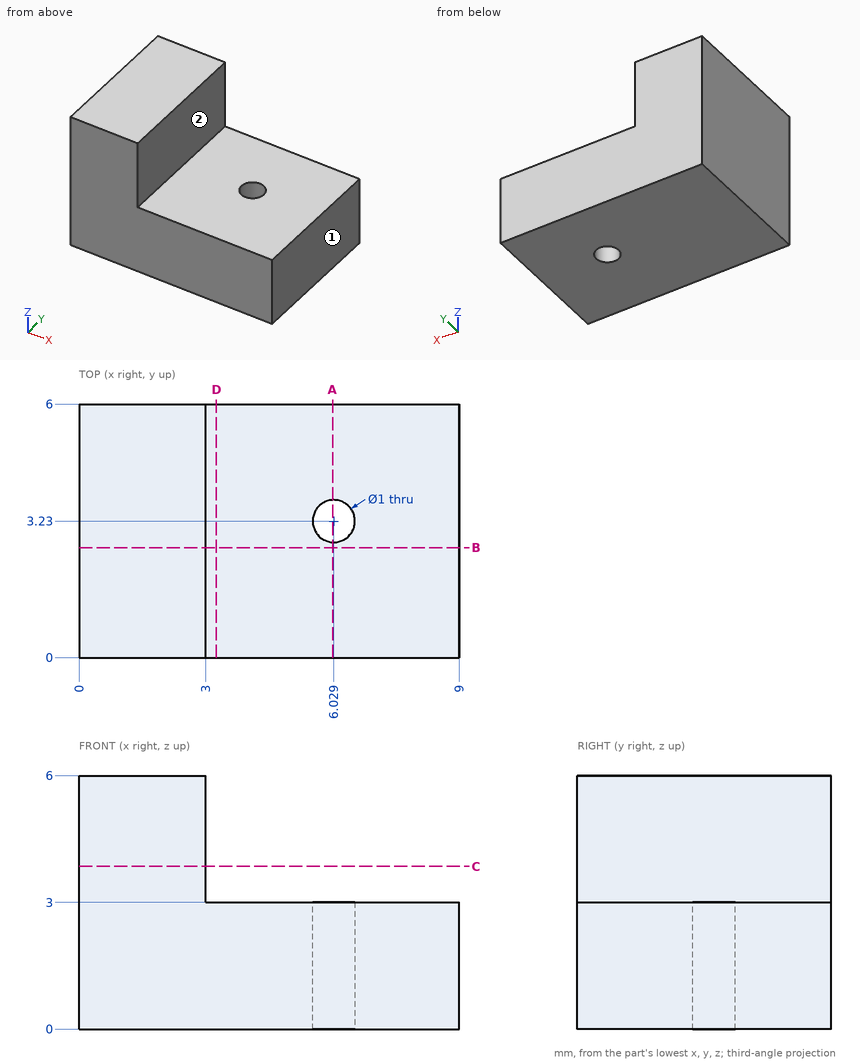
For this review, use the dimensioned drawing (mm, ordinates from the lowest corner) and the shaded views. A direction names the side the tool comes from. Round coordinates to 2 decimals unless told otherwise and drop trailing zeros. Order: outer loops, then holes, each group sorted by start corner. A loop starts at its lowest first (then second) coordinate and runs counter-clockwise, first axis right, second up. Notation, with made-up numbers: (62, -1) -> (116, -1) arc R26 cw to (116, 19) -> close; hole circle Ø9 at (-30, -18). An arc over 180 degrees is marked (long way). Write item = value, one per line. Start each with the question number.
Item 1: Clearance check with a flat-ended pin moving along its axis: pin 1 Ø3 at (x, y) = (6, 2.5) entering from +Z. State where the tip first meets the part, or that it passes through.
Item 2: For the marked faces 1 and 2, list the 3-axis set-ups (+Z, -Z, +X, -X, +Y, -Y) from which the entire face can be reached by the end or side of a thin tool; tool diameter is ignored.
Item 3: Consider section A-A on x = 6. Write out the cut boundary in (y, z).
Item 4: For line 1 along X through (y, z) = (4.2, 3.6); line 2 along X through (y, z) = (3.5, 0.6), list the stretches that pass through material, from the lowest coordinate up.
Item 5: Consider section B-B on y = 2.6. Write out the cut boundary in (x, z), plus the area to 3 significant figures.
Item 6: Consider section D-D on x = 3.25. Write out the cut boundary in (y, z).
Item 7: Consider section C-C on z = 3.85. Write out the cut boundary in (x, y), plus the area to 3 significant figures.
Conclusion:
q1.pin_1 = 3
q2.face_1 = +Z, -Z, +X, +Y, -Y
q2.face_2 = +Z, +X, +Y, -Y
q3.outline = (0, 0) -> (2.73, 0) -> (2.73, 3) -> (0, 3) -> close; (3.73, 0) -> (6, 0) -> (6, 3) -> (3.73, 3) -> close
q4.line_1 = 0 to 3
q4.line_2 = 0 to 5.61, 6.45 to 9
q5.outline = (0, 0) -> (9, 0) -> (9, 3) -> (3, 3) -> (3, 6) -> (0, 6) -> close
q5.area = 36.0 mm2
q6.outline = (0, 0) -> (6, 0) -> (6, 3) -> (0, 3) -> close
q7.outline = (0, 0) -> (3, 0) -> (3, 6) -> (0, 6) -> close
q7.area = 18.0 mm2
